Input: part model. Units: mm. Frame: model coordinates. A direction names the side the tool comes from. Round coordinates to 2 decimals unless told otherwise and drop trailing zeros. Order: outer loops, then holes, each group sorted by start corner. A loop starts at its lowest first (then second) coordinate and runs counter-clockwise, first axis right, second up. Notation, with made-up numbers: (61, 63) -> (77, 63) arc R17 cw to (77, 77) -> close; hole circle Ø7 at (-35.5, 56.25). An arc over 180 degrees is marked (long way). Use a Markdown table: item, result.
from build123d import *
from build123d.topology import SkipClean

# Parameters (mm, degrees)
SKETCH1_R      = 3.1
EXTRUDE1_DEPTH = 1.5
SKETCH2_R      = 4.1
SKETCH2_R_2    = 1.5
EXTRUDE2_DEPTH = 1.5
EXTRUDE3_START = 7.8
SKETCH3_R      = 2.5
EXTRUDE3_DEPTH = 7.8
SKETCH4_R      = 1.4
EXTRUDE4_DEPTH = 1.6
SKETCH5_R      = 8
EXTRUDE5_DEPTH = 31.443100442
SKETCH6_R      = 10
SKETCH6_R_2    = 8
EXTRUDE6_DEPTH = 5


with BuildPart() as part:
    # Sketch1 → Extrude1 (new body)
    with BuildSketch(Plane.XY):
        with BuildLine():
            Line((-11.4, 15.5), (11.4, 15.5))
            ThreePointArc((11.4, 15.5), (15.5, 19.6), (19.6, 15.5))
            Line((19.6, 15.5), (19.6, 3.03001766))
            ThreePointArc((19.6, 3.03001766), (21.313431552, 0.656979507), (19.6, -1.716058647))
            Line((19.6, -1.716058647), (19.6, -15.5))
            ThreePointArc((19.6, -15.5), (15.5, -19.6), (11.4, -15.5))
            Line((11.4, -15.5), (-11.4, -15.5))
            ThreePointArc((-11.4, -15.5), (-15.5, -19.6), (-19.6, -15.5))
            Line((-19.6, -15.5), (-19.6, -3.03001766))
            ThreePointArc((-19.6, -3.03001766), (-21.313431552, -0.656979507), (-19.6, 1.716058647))
            Line((-19.6, 1.716058647), (-19.6, 15.5))
            ThreePointArc((-19.6, 15.5), (-15.5, 19.6), (-11.4, 15.5))
        make_face()
        with Locations((15.5, -15.5)):
            Circle(SKETCH1_R, mode=Mode.SUBTRACT)
        with Locations((-15.5, 15.5)):
            Circle(SKETCH1_R, mode=Mode.SUBTRACT)
        with BuildLine():
            Line((-12.40645834, -15.3), (-18.59354166, -15.3))
            ThreePointArc((-18.59354166, -15.3), (-15.5, -18.6), (-12.40645834, -15.3))
        make_face(mode=Mode.SUBTRACT)
        with BuildLine():
            Line((18.59354166, 15.3), (12.40645834, 15.3))
            ThreePointArc((12.40645834, 15.3), (15.5, 18.6), (18.59354166, 15.3))
        make_face(mode=Mode.SUBTRACT)
    extrude(amount=EXTRUDE1_DEPTH)

    # Sketch2 → Extrude2 (add)
    # profile 1 of 4: a face of its own
    with SkipClean():  # the faces are left unmerged after this step: merging them gives an invalid solid
        with BuildSketch(Plane.XY.offset(1.5)):
            with Locations((-15.5, 15.5)):
                Circle(SKETCH2_R)
            with Locations((-15.5, 15.5)):
                Circle(SKETCH2_R_2, mode=Mode.SUBTRACT)
        # profile 2 of 4: a face of its own
        with BuildSketch(Plane.XY.offset(1.5)):
            with Locations((15.5, 15.5)):
                Circle(SKETCH2_R)
        # profile 3 of 4: a face of its own
        with BuildSketch(Plane.XY.offset(1.5)):
            with Locations((15.5, -15.5)):
                Circle(SKETCH2_R)
            with Locations((15.5, -15.5)):
                Circle(SKETCH2_R_2, mode=Mode.SUBTRACT)
        # profile 4 of 4: a face of its own
        with BuildSketch(Plane.XY.offset(1.5)):
            with Locations((-15.5, -15.5)):
                Circle(SKETCH2_R)
        extrude(amount=EXTRUDE2_DEPTH)
    add(part.part.scale(1), mode=Mode.REPLACE)  # the faces are merged on a copy

    # Sketch3 → Extrude3 (add)
    with BuildSketch(Plane(origin=(0, 0, 0), x_dir=(-1, 0, 0), z_dir=(0, 0, -1)).offset(EXTRUDE3_START)):
        with Locations((18.813431552, -0.656979507)):
            Circle(SKETCH3_R)
        with Locations((-18.813431552, 0.656979507)):
            Circle(SKETCH3_R)
    extrude(amount=-EXTRUDE3_DEPTH)

    # Sketch4 → Extrude4 (add)
    with BuildSketch(Plane(origin=(0, 0, -7.8), x_dir=(-1, 0, 0), z_dir=(0, 0, -1))):
        with Locations((-18.813431552, 0.656979507)):
            Circle(SKETCH4_R)
        with Locations((18.813431552, -0.656979507)):
            Circle(SKETCH4_R)
    extrude(amount=EXTRUDE4_DEPTH)

    # Sketch5 → Extrude5 (cut, through all)
    with BuildSketch(Plane(origin=(0, 0, 0), x_dir=(-1, 0, 0), z_dir=(0, 0, -1))):
        Circle(SKETCH5_R)
    extrude(amount=-EXTRUDE5_DEPTH, mode=Mode.SUBTRACT)

    # Sketch6 → Extrude6 (add)
    with SkipClean():  # the faces are left unmerged after this step: merging them gives an invalid solid
        with BuildSketch(Plane.XY.offset(1.5)):
            with Locations(Location((0, 0, 0), (0, 0, 180))):
                Circle(SKETCH6_R)
            with Locations(Location((0, 0, 0), (0, 0, 180))):
                Circle(SKETCH6_R_2, mode=Mode.SUBTRACT)
        extrude(amount=EXTRUDE6_DEPTH)


solid = part.part
1) Cut plane B-B on y = 0. Return loops of the section in (x, z), and give its area (3 significant figures).
Results found:
| item | result |
|---|---|
| outline | (-21.23, -7.8) -> (-20.05, -7.8) -> (-20.05, -9.4) -> (-17.58, -9.4) -> (-17.58, -7.8) -> (-16.4, -7.8) -> (-16.4, 0) -> (-8, 0) -> (-8, 6.5) -> (-10, 6.5) -> (-10, 1.5) -> (-21.23, 1.5) -> close; (8, 0) -> (16.4, 0) -> (16.4, -7.8) -> (17.58, -7.8) -> (17.58, -9.4) -> (20.05, -9.4) -> (20.05, -7.8) -> (21.23, -7.8) -> (21.23, 1.5) -> (10, 1.5) -> (10, 6.5) -> (8, 6.5) -> close |
| area | 143 mm² |
2) Cut plane A-A on x = -15.5. Return loops of the section in (y, z), and give its area (4 significant figures).
Results found:
| item | result |
|---|---|
| outline | (-19.6, 0) -> (-18.6, 0) -> (-18.6, 1.5) -> (-15.3, 1.5) -> (-15.3, 0) -> (12.4, 0) -> (12.4, 1.5) -> (14, 1.5) -> (14, 3) -> (11.4, 3) -> (11.4, 1.5) -> (-11.4, 1.5) -> (-11.4, 3) -> (-19.6, 3) -> close; (17, 1.5) -> (18.6, 1.5) -> (18.6, 0) -> (19.6, 0) -> (19.6, 3) -> (17, 3) -> close |
| area | 64.65 mm² |
3) Pull-direction query (X, two-part tool) for faces 4 (the cylindrical face through (10, 0, 4)), 5 (the flat face through (0, -8.2, 6.5)), 6 (the flat face through (15, 17, 1.5)); classes: +X half, -X half, draft (parallel to the pull), parting line (faces both ways), or undercut.
Results found:
| item | result |
|---|---|
| face 4 | parting line |
| face 5 | draft |
| face 6 | undercut |
4) Set-up query: faces 1 (the cylindrical face through (15.4, 18.6, 0.7)), 2 (the flat face through (0, -15.5, 1)), 3 (the flat face through (19.6, 9, 1)). Return all of +Z, -Z, +X, -X, +Y, -Y with unobstructed straight access to the full face (end or side cutting, diameter ignored); none if empty.
Results found:
| item | result |
|---|---|
| face 1 | -Z |
| face 2 | +Z, -Z, -Y |
| face 3 | +Z, -Z, +X, +Y |
5) Cut plane C-C on x = 6.5. Return loops of the section in (y, z), and give its area (3 significant figures).
Results found:
| item | result |
|---|---|
| outline | (-15.5, 0) -> (-4.66, 0) -> (-4.66, 6.5) -> (-7.6, 6.5) -> (-7.6, 1.5) -> (-15.5, 1.5) -> close; (4.66, 0) -> (15.5, 0) -> (15.5, 1.5) -> (7.6, 1.5) -> (7.6, 6.5) -> (4.66, 6.5) -> close |
| area | 61.9 mm² |
6) Line query: L1, parallel to Y at x = -15.5, z = 1.1; L2, parallel to Y at x = 0, z = 1; L3, parallel to Y at x = 15.5, z = 1.15. Output: solid intervals per line, ascending. Write a range as [from, to].
Results found:
| item | result |
|---|---|
| L1 | y = [-19.6, -18.6], [-15.3, 12.4], [18.6, 19.6] |
| L2 | y = [-15.5, -8], [8, 15.5] |
| L3 | y = [-19.6, -18.6], [-12.4, 15.3], [18.6, 19.6] |
7) Cut plane D-D on y = -7.5. Return loops of the section in (x, z), and give its area (3 significant figures).
Results found:
| item | result |
|---|---|
| outline | (-19.6, 0) -> (-2.78, 0) -> (-2.78, 6.5) -> (-6.61, 6.5) -> (-6.61, 1.5) -> (-19.6, 1.5) -> close; (2.78, 0) -> (19.6, 0) -> (19.6, 1.5) -> (6.61, 1.5) -> (6.61, 6.5) -> (2.78, 6.5) -> close |
| area | 88.8 mm² |
8) Pin query (flat end, axial travel): pin 1 Ø3.5 at (x, y) = (-15.5, 15.5) entering from +Z; pin 2 Ø21 at (x, y) = (0, 0) entering from +Z; pin 3 Ø3 at (y, z) = (3, -1) entering from -X; pin 4 Ø8 at (x, y) = (15.5, -15.5) entering from -Z. Return the tip coordinate at first contact, or that it passes through.
Results found:
| item | result |
|---|---|
| pin 1 | stops at z = 3 |
| pin 2 | stops at z = 6.5 |
| pin 3 | stops at x = -20.08 |
| pin 4 | stops at z = 0 |
